Autodesk Inventor part; units mm, degrees
ref_plane "YZ Plane" through (0, 0, 0) normal (1, 0, 0) x (0, 1, 0)
ref_plane "XZ Plane" through (0, 0, 0) normal (0, 1, 0) x (-1, 0, 0)
ref_plane "XY Plane" through (0, 0, 0) normal (0, 0, 1) x (1, 0, 0)
sketch "スケッチ1" plane through (0, 0, 0) normal (0, 0, 1) x (1, 0, 0)
  circle A0 centre (0, 0) radius 2.75
  dimension "d0" = 5.5
extrude "押し出し1" add sketch "スケッチ1" along normal blind 2
fillet "フィレット1" radius 1 1 edges at (-2.75, 0, 2)
sketch "スケッチ2" plane through (0, 0, 0) normal (0, 0, -1) x (-1, 0, 0)
  circle A0 centre (0, 0) radius 1.5
  dimension "d4" = 3
extrude "押し出し2" add sketch "スケッチ2" along normal blind 5
thread "ねじ1"
properties part number "Screw_5mm" material "真鍮"
For this review, take the finished solid that the model builds, in its own axes (mm). A direction names the side the tool comes from. Round coordinates to 2 decimals unless told otherwise and drop trailing zeros. Write each loop counter-clockwise with the first axis right and the second up, starting at its lowest first coordinate (ties: lowest second). Pieces come first, ordered by that corner, then holes. Notation, with made-up numbers: (58.25, -29.75) - (86.25, -29.75) arc R23 cw to (86.25, -6.75) - close; hole circle Ø4 at (-23, 75). An arc over 180 degrees is marked (long way). Use CSV: the item, a comma, the result in double quotes.
1) Add section C-C on z = -1.5. Write out the cut boundary in (x, y), and give its area (3 significant figures).
Conclusion:
outline,"circle Ø3 at (0, 0)"
area,"7.07 mm^2"
2) Add section D-D on z = 0.25. Write out the cut boundary in (x, y), and give its area (3 significant figures).
Conclusion:
outline,"circle Ø5.5 at (0, 0)"
area,"23.8 mm^2"
3) For faces 1 (the flat face through (1.2, -1.2, 0)), 2 (the flat face through (0, 0, 2)), list the 3-axis set-ups (+Z, -Z, +X, -X, +Y, -Y) from which the entire face can be reached by the end or side of a thin tool; tool diameter is ignored.
Conclusion:
face 1,"-Z"
face 2,"+Z, +X, -X, +Y, -Y"
4) Wall thickness on line 1 along X through (y, z) = (2.05, 1.5); line 2 along X through (y, z) = (-0.65, -4); line 3 along Z through (x, y) = (-0.5, -2.35): over which ranges is each line inside the solid? List them lowest first. Write a range as from..to.
Conclusion:
line 1,"x = -1.63..1.63"
line 2,"x = -1.35..1.35"
line 3,"z = 0..1.76"
5) Add section A-A on y = 0. Write out the cut boundary in (x, z).
Conclusion:
outline,"(-2.75, 0) - (-1.5, 0) - (-1.5, -5) - (1.5, -5) - (1.5, 0) - (2.75, 0) - (2.75, 1) arc R1 ccw to (1.75, 2) - (-1.75, 2) arc R1 ccw to (-2.75, 1) - close"
